For this review, use the dimensioned drawing (mm, ordinates from the lowest corner) and the shaded views. Coordinates: 2 decimals unless noted, no trailing zeros. Loops run counter-clockwise (first coordinate to the right, second up) from the corner with the lowest first, then second, coordinate; pieces in that order, holes last.
1. Take a section at A-A, the plane z = 8.5. State the section outline as (x, y) points.
2. Take a section at D-D, the plane z = 51.5. State the section outline as (x, y) points.
3. Clearance check with flat-ended pins moving along their axes: P1, Ø1.4, axis at y = 1.5, z = 30, coming from the +X side; P2, Ø2.5, axis at y = 3, z = 31.5, coming from the -X side. State where each tip first meets the part, or that it passes through.
4. Take a section at C-C, the plane x = 8.5. State the section outline as (y, z) points, then the cut area to 3 significant figures.
5. Take a section at B-B, the plane y = 2.9. State the section outline as (x, z) points.
6. Mouldability with a two-part tool opening along X and no side actions: class the marked faces 1, 2, 3 and 4 as pulls with the +X half, pulls with the -X half, needs draft (parallel to the pull), parting line crosses it, or undercut.
7. To check wall thickness, follow probe 1 along X at (y, z) = (1.8, 8.5); probe 2 along X at (y, z) = (3.05, 39.5); probe 3 along X at (y, z) = (4, 7.5). State the ranges of each line that lie inside material, in increasing order.
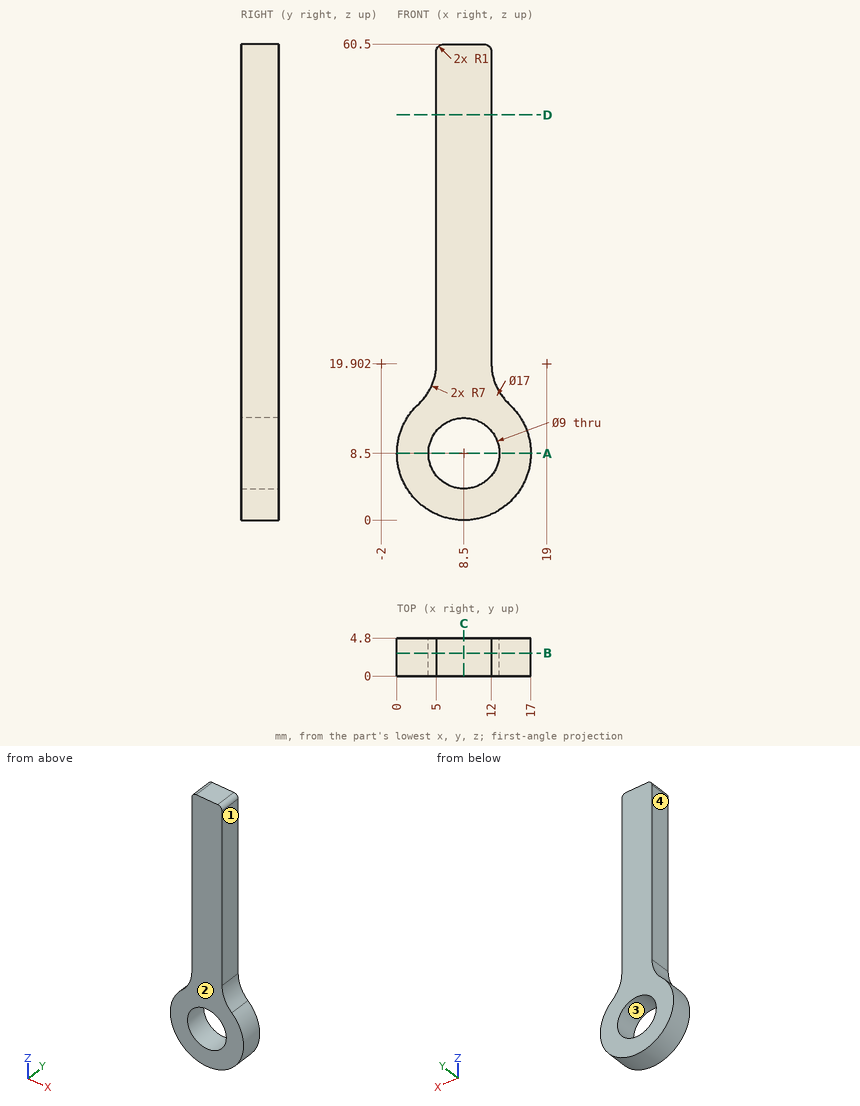
Results list:
1. outline: (0, 0) - (4, 0) - (4, 4.8) - (0, 4.8) - close; (13, 0) - (17, 0) - (17, 4.8) - (13, 4.8) - close
2. outline: (5, 0) - (12, 0) - (12, 4.8) - (5, 4.8) - close
3. P1: stops at x = 12
3. P2: stops at x = 5
4. outline: (0, 0) - (4.8, 0) - (4.8, 4) - (0, 4) - close; (0, 13) - (4.8, 13) - (4.8, 60.5) - (0, 60.5) - close
4. area: 247 mm2
5. outline: (2.74, 14.75) arc R8.5 ccw (long way) to (14.26, 14.75) arc R7 cw to (12, 19.9) - (12, 59.5) arc R1 ccw to (11, 60.5) - (6, 60.5) arc R1 ccw to (5, 59.5) - (5, 19.9) arc R7 cw to start; hole circle Ø9 at (8.5, 8.5)
6. face 1: pulls with the +X half
6. face 2: needs draft
6. face 3: undercut
6. face 4: pulls with the -X half
7. probe 1: x = 0 to 4, 13 to 17
7. probe 2: x = 5 to 12
7. probe 3: x = 0.06 to 4.11, 12.89 to 16.94
